from build123d import *

# Parameters (mm, degrees)
SKETCH1_W           = 647.7
SKETCH1_H           = 50.8
SKETCH1_R           = 12.7
BOSS_EXTRUDE1_DEPTH = 6.35


with BuildPart() as part:
    # Sketch1 → Boss-Extrude1 (new body)
    with BuildSketch(Plane(origin=(0, 0, 0), x_dir=(0, 0, -1), z_dir=(1, 0, 0))):
        with Locations((323.85, 25.4)):
            Rectangle(SKETCH1_W, SKETCH1_H)
        with Locations((23.370832151, 25.4)):
            Circle(SKETCH1_R, mode=Mode.SUBTRACT)
        with Locations((56.390832151, 25.4)):
            Circle(SKETCH1_R, mode=Mode.SUBTRACT)
        with Locations((89.410832151, 25.4)):
            Circle(SKETCH1_R, mode=Mode.SUBTRACT)
        with Locations((122.430832151, 25.4)):
            Circle(SKETCH1_R, mode=Mode.SUBTRACT)
        with Locations((155.450832151, 25.4)):
            Circle(SKETCH1_R, mode=Mode.SUBTRACT)
        with Locations((188.470832151, 25.4)):
            Circle(SKETCH1_R, mode=Mode.SUBTRACT)
        with Locations((221.490832151, 25.4)):
            Circle(SKETCH1_R, mode=Mode.SUBTRACT)
        with Locations((254.510832151, 25.4)):
            Circle(SKETCH1_R, mode=Mode.SUBTRACT)
        with Locations((287.530832151, 25.4)):
            Circle(SKETCH1_R, mode=Mode.SUBTRACT)
        with Locations((320.550832151, 25.4)):
            Circle(SKETCH1_R, mode=Mode.SUBTRACT)
        with Locations((353.570832151, 25.4)):
            Circle(SKETCH1_R, mode=Mode.SUBTRACT)
        with Locations((386.590832151, 25.4)):
            Circle(SKETCH1_R, mode=Mode.SUBTRACT)
        with Locations((419.610832151, 25.4)):
            Circle(SKETCH1_R, mode=Mode.SUBTRACT)
        with Locations((452.630832151, 25.4)):
            Circle(SKETCH1_R, mode=Mode.SUBTRACT)
        with Locations((485.650832151, 25.4)):
            Circle(SKETCH1_R, mode=Mode.SUBTRACT)
        with Locations((518.670832151, 25.4)):
            Circle(SKETCH1_R, mode=Mode.SUBTRACT)
        with Locations((551.690832151, 25.4)):
            Circle(SKETCH1_R, mode=Mode.SUBTRACT)
        with Locations((584.710832151, 25.4)):
            Circle(SKETCH1_R, mode=Mode.SUBTRACT)
        with Locations((617.730832151, 25.4)):
            Circle(SKETCH1_R, mode=Mode.SUBTRACT)
    extrude(amount=BOSS_EXTRUDE1_DEPTH)


solid = part.part
The model under review builds one solid part; all positions refer to its coordinate system, in mm. Give positions to 0.01 mm unless a question says otherwise; leave off trailing zeros. Loops run counter-clockwise (first coordinate to the right, second up) from the corner with the lowest first, then second, coordinate; pieces in that order, holes last. Notation, with made-up numbers: (41, 57.5) -> (56, 57.5) arc R30 cw to (56, 89.5) -> close; hole circle Ø2 at (-8.5, -15.75). An arc over 180 degrees is marked (long way). Put each result on its own line as item: value. Start each with the question number.
1. We need section B-B on z = -57.5. State the section outline as (x, y) points, then the cut area to 3 significant figures.
2. Mouldability with a two-part tool opening along Y and no side actions: class faces 1 (the face through (6.35, 9, -319)), 2 (the face through (3.131, 29.215, -266.624)) as released by +Y, released by -Y, zero draft, split by the parting line, or undercut.
3. Wall thickness on probe 1 along Y at (x, z) = (2.25, -618); probe 2 along Y at (x, z) = (1.25, -497): over which ranges is each line inside the solid? List them lowest first.
4. We need section A-A on x = 4.5. State how many separate pieces and enclosed holes the cut face has, then the cut area to 3 significant figures.
5. We need section D-D on z = -183. State the section outline as (x, y) points, then the cut area to 3 significant figures.
Determined:
1. outline: (0, 0) -> (6.35, 0) -> (6.35, 12.75) -> (0, 12.75) -> close; (0, 38.05) -> (6.35, 38.05) -> (6.35, 50.8) -> (0, 50.8) -> close
1. area: 162 mm^2
2. face 1: zero draft
2. face 2: undercut
3. probe 1: 0 to 12.7, 38.1 to 50.8
3. probe 2: 0 to 19.7, 31.1 to 50.8
4. separate pieces: 1
4. enclosed holes: 19
4. area: 23,300 mm^2
5. outline: (0, 0) -> (6.35, 0) -> (6.35, 13.94) -> (0, 13.94) -> close; (0, 36.86) -> (6.35, 36.86) -> (6.35, 50.8) -> (0, 50.8) -> close
5. area: 177 mm^2
